Could you check a few things on this model? Use its own coordinates, in mm. A direction names the side the tool comes from. Round coordinates to 2 decimals unless told otherwise and drop trailing zeros. Write each loop counter-clockwise with the first axis right and the second up, starting at its lowest first coordinate (ties: lowest second). Pieces come first, ordered by that corner, then holes. Notation, with made-up numbers: (37, 4.25) -> (45, 4.25) arc R25 ccw to (45, 35.25) -> close; hole circle Ø1 at (37, -21.5). An arc over 180 degrees is marked (long way). Answer in a Markdown table with one row per item.
from build123d import *

# Parameters (mm, degrees)
F0_W     = 145
F0_H     = 30
F1_DEPTH = 3
F2_W     = 10
F2_H     = 3
F3_DEPTH = 25


with BuildPart() as f1:
    # F0 (on Front) → F1 (new body)
    with BuildSketch(Plane.XZ):
        Rectangle(F0_W, F0_H)
    extrude(amount=F1_DEPTH)

    # F2 (on face) → F3 (cut)
    with BuildSketch(Plane.XZ.offset(3)):
        with Locations((-70, -13.5)):
            Rectangle(F2_W, F2_H)
        with Locations((-70, 13.5)):
            Rectangle(F2_W, F2_H)
        with Locations((-50, -13.5)):
            Rectangle(F2_W, F2_H)
        with Locations((-50, 13.5)):
            Rectangle(F2_W, F2_H)
        with Locations((-30, -13.5)):
            Rectangle(F2_W, F2_H)
        with Locations((-30, 13.5)):
            Rectangle(F2_W, F2_H)
        with Locations((-10, -13.5)):
            Rectangle(F2_W, F2_H)
        with Locations((-10, 13.5)):
            Rectangle(F2_W, F2_H)
        with Locations((10, -13.5)):
            Rectangle(F2_W, F2_H)
        with Locations((10, 13.5)):
            Rectangle(F2_W, F2_H)
        with Locations((30, -13.5)):
            Rectangle(F2_W, F2_H)
        with Locations((30, 13.5)):
            Rectangle(F2_W, F2_H)
        with Locations((50, -13.5)):
            Rectangle(F2_W, F2_H)
        with Locations((50, 13.5)):
            Rectangle(F2_W, F2_H)
        with Locations((70, -13.5)):
            Rectangle(F2_W, F2_H)
        with Locations((70, 13.5)):
            Rectangle(F2_W, F2_H)
    extrude(amount=-F3_DEPTH, mode=Mode.SUBTRACT)


solid = f1.part
1) For pin 1 (0.9 mm diameter, centred on x = -51, y = -1, fed in from -Z); pin 2 (0.9 mm diameter, centred on y = -1.5, z = -14, fed in from -X); pin 3 (0.9 mm diameter, centred on y = -1.5, z = 14, fed in from +X); pin 4 (3 mm diameter, centred on x = -46, z = 7, fed in from +Y), each with a flat end and sliding along its axis, tell me the tip position at first contact or that it passes through.
Findings:
| item | result |
|---|---|
| pin 1 | stops at z = -12 |
| pin 2 | stops at x = -65 |
| pin 3 | stops at x = 65 |
| pin 4 | stops at y = 0 |
2) For faces 5 (the face through (40, -1, 15)), 6 (the face through (-35, -2, 13)), 7 (the face through (-35, -2, -14)), 8 (the face through (69, -2, 12)), which set-ups out of +Z, -Z, +X, -X, +Y, -Y let a thin tool reach every point of the face, with its end or its side?
Findings:
| item | result |
|---|---|
| face 5 | +Z, +X, -X, +Y, -Y |
| face 6 | +Z, +Y, -Y |
| face 7 | -Z, +Y, -Y |
| face 8 | +Z, +X, +Y, -Y |
3) Please list where this line runs through material, in increasing order: line 1 (Z direction, x = -52.5, y = -2.4).
Findings:
| item | result |
|---|---|
| line 1 | z = -12 to 12 |
4) Imagine slicing it at A-A, the plane x = -10.5. Please give me the cut outline in (y, z).
Findings:
| item | result |
|---|---|
| outline | (-3, -12) -> (0, -12) -> (0, 12) -> (-3, 12) -> close |
5) Thinking about a two-plate mould opening in X: for faces 1 (the face through (40, -1, -15)), 2 (the face through (65, -2, -14)), 3 (the face through (55, -2, -14)), 4 (the face through (50, -2, -12)), which applies, +X half, -X half, draft (parallel to the pull), parting line (faces both ways), or undercut?
Findings:
| item | result |
|---|---|
| face 1 | draft |
| face 2 | +X half |
| face 3 | undercut |
| face 4 | undercut |
